For this review, use the dimensioned drawing (mm, ordinates from the lowest corner) and the shaded views. Round coordinates to 2 decimals unless told otherwise and drop trailing zeros. Write each loop counter-clockwise with the first axis right and the second up, starting at its lowest first coordinate (ties: lowest second). Pieces come first, ordered by that corner, then holes.
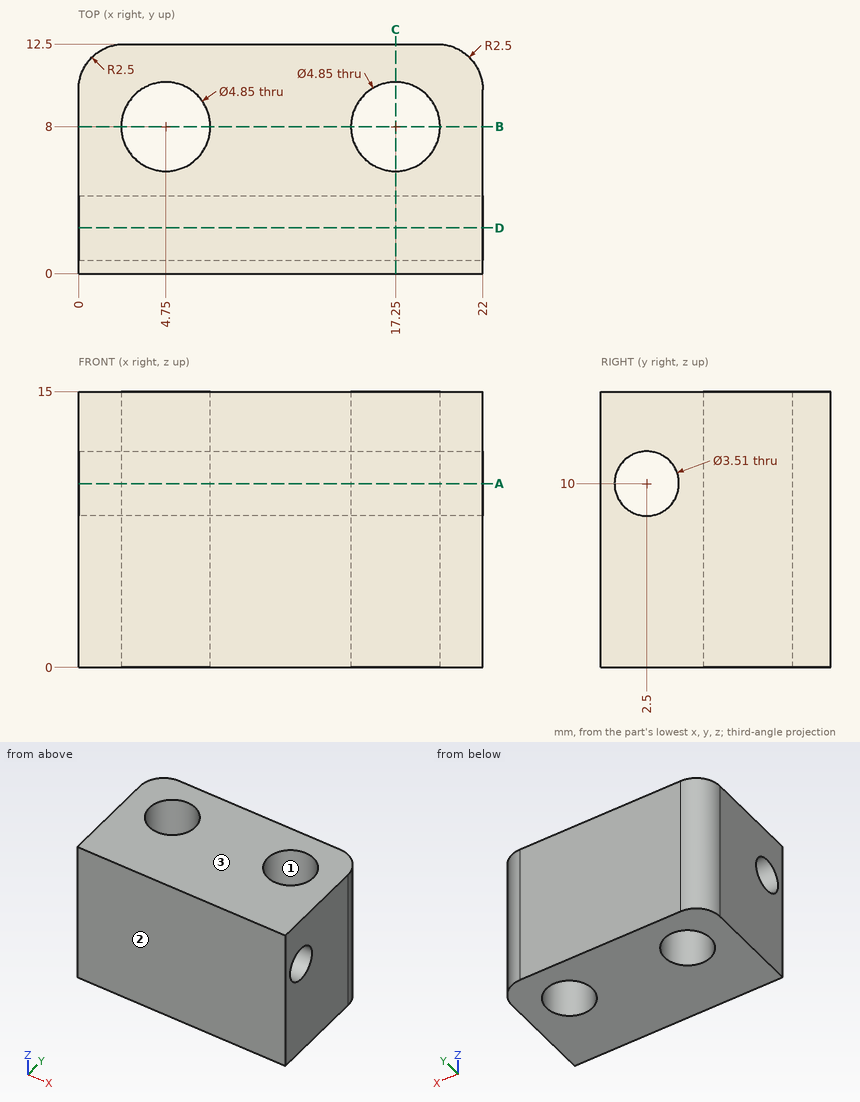
1) The part is to be moulded in two halves that separate along Y. For the marked faces 1, 2 and 3, say which applies: pulls with the +Y half, pulls with the -Y half, needs draft (parallel to the pull), parting line crosses it, or undercut.
2) For line 1 along Y through (x, z) = (4.75, 10) (3 decimals); line 2 along Y through (x, z) = (18.25, 10.75); line 3 along X through (y, z) = (8.75, 9.25), list the stretches that pass through material, from the lowest coordinate up.
3) Add section B-B on y = 8. State the section outline as (x, z) points (3 decimals).
4) Add section A-A on z = 10. State the section outline as (x, y) points (3 decimals), and give its area (3 significant figures).
5) Add section C-C on x = 17.25. State the section outline as (y, z) points (3 decimals), and give its area (3 significant figures).
6) For P1, Ø1.5, axis at x = 5, z = 6.5, coming from the -Y side, flat-tipped, find the tip position at first contact; note if it passes through.
7) Add section D-D on y = 2.5. State the section outline as (x, z) points (3 decimals), and give its area (3 significant figures).
Computed:
1. face 1: undercut
1. face 2: pulls with the -Y half
1. face 3: needs draft
2. line 1: y = 0 to 0.745, 4.255 to 5.575, 10.425 to 12.5
2. line 2: y = 0 to 0.91, 4.09 to 5.79, 10.21 to 12.5
2. line 3: x = 0 to 2.44, 7.06 to 14.94, 19.56 to 22
3. outline: (0, 0) - (2.325, 0) - (2.325, 15) - (0, 15) - close; (7.175, 0) - (14.825, 0) - (14.825, 15) - (7.175, 15) - close; (19.675, 0) - (22, 0) - (22, 15) - (19.675, 15) - close
4. outline: (0, 0) - (22, 0) - (22, 0.745) - (0, 0.745) - close; (0, 4.255) - (22, 4.255) - (22, 10) arc R2.5 ccw to (19.5, 12.5) - (2.5, 12.5) arc R2.5 ccw to (0, 10) - close; hole circle Ø4.85 at (4.75, 8); hole circle Ø4.85 at (17.25, 8)
4. area: 158 mm2
5. outline: (0, 0) - (5.575, 0) - (5.575, 15) - (0, 15) - close; (10.425, 0) - (12.5, 0) - (12.5, 15) - (10.425, 15) - close; hole circle Ø3.51 at (2.5, 10)
5. area: 105 mm2
6. P1: stops at y = 0
7. outline: (0, 0) - (22, 0) - (22, 8.245) - (0, 8.245) - close; (0, 11.755) - (22, 11.755) - (22, 15) - (0, 15) - close
7. area: 253 mm2
